Verification items for the finished model (mm, model axes). Face numbers are marked on the shaded views. A direction names the side the tool comes from. Round coordinates to 2 decimals unless told otherwise and drop trailing zeros. Order: outer loops, then holes, each group sorted by start corner. A loop starts at its lowest first (then second) coordinate and runs counter-clockwise, first axis right, second up.
```python
from build123d import *

# Parameters (mm, degrees)
F0_W     = 19.05
F0_H     = 69.85
F1_ANGLE = -270
F2_R     = 3.048
F3_W     = 34.798
F3_H     = 35.052
F4_ANGLE = 270
F5_R     = 3.048
F6_R     = 19.05
F7_DEPTH = 53.849
F8_R     = 6.35
F9_DEPTH = 19.051


with BuildPart() as f1:
    # F0 (on Right) → F1 (revolve)
    with BuildSketch(Plane.YZ):
        with Locations((9.525, 34.925)):
            Rectangle(F0_W, F0_H)
    revolve(axis=Axis((0, 9.525, 0), (0, 1, 0)), revolution_arc=F1_ANGLE)

    # F2
    f2_edges = [f1.edges().sort_by_distance(p)[0] for p in [
        (-49.391409, 0, -49.391409),
    ]]
    fillet(f2_edges, radius=F2_R)

    # F3 (on Right) → F4 (revolve)
    with BuildSketch(Plane.YZ):
        with Locations((-17.399, 17.526)):
            Rectangle(F3_W, F3_H)
    revolve(axis=Axis((0, -17.399, 0), (0, -1, 0)), revolution_arc=F4_ANGLE)

    # F5
    f5_edges = [f1.edges().sort_by_distance(p)[0] for p in [
        (-24.785507, -34.798, -24.785507),
        (-24.785507, 0, -24.785507),
    ]]
    fillet(f5_edges, radius=F5_R)

    # F6 (on face) → F7 (cut, through all)
    with BuildSketch(Plane.XZ.offset(34.798)):
        Circle(F6_R)
    extrude(amount=-F7_DEPTH, mode=Mode.SUBTRACT)

    # F8 (on Front) → F9 (cut, through all)
    with BuildSketch(Plane.XZ):
        with Locations((0, 53.848)):
            Circle(F8_R)
        with Locations((-53.848, 0)):
            Circle(F8_R)
        with Locations((0, -53.848)):
            Circle(F8_R)
        with Locations((53.848, 0)):
            Circle(F8_R)
    extrude(amount=-F9_DEPTH, mode=Mode.SUBTRACT)


solid = f1.part
```
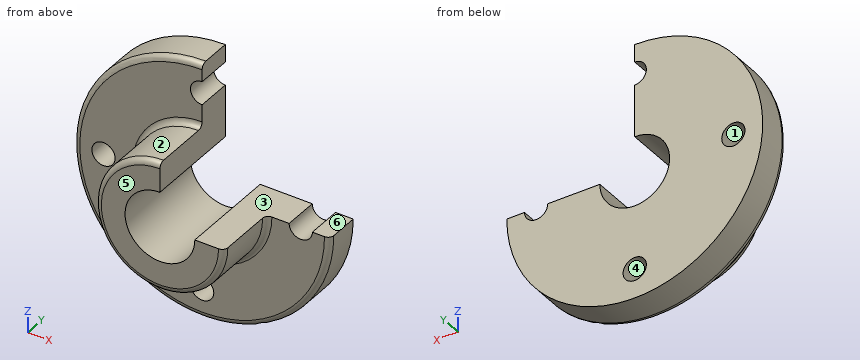
1) Go/stop test with flat-tipped pins: pin 1 Ø2 at (x, y) = (28.5, -7.5) entering from +Z; pin 2 Ø5 at (y, z) = (7, -34) entering from -X; pin 3 Ø5 at (y, z) = (10.5, 65.5) entering from +X. Record where each tip stops, or that it passes through.
2) Scan lines: probe 1 along X at (y, z) = (16.5, -2); probe 2 along Y at (x, z) = (28.5, -32); probe 3 along X at (y, z) = (-2.5, -10). Record each from-to range of solid material in increasing order.
3) Sectioned sample at A-A on y = 7.5. Record the cut outline in (x, z), then the cut area to 3 significant figures.
4) Sectioned sample at B-B on y = -23. Record the cut outline in (x, z), then the cut area to 3 significant figures.
5) Draft check along Z on the marked faces 4, 5 and 6. Enter one of: released by +Z, released by -Z, zero draft, split by the parting line, or undercut.
6) Tool access check on the marked faces 1, 2 and 3. Record the directions out of +Z, -Z, +X, -X, +Y, -Y that give a thin tool (end or side, any length) a straight path to the whole face; none if there is none.
Returned:
1. pin 1: stops at z = 0
1. pin 2: stops at x = -62.34
1. pin 3: stops at x = 0
2. probe 1: x = -69.82 to -59.87, -47.82 to -18.94, 18.94 to 47.82, 59.87 to 69.82
2. probe 2: y = 0 to 19.05
2. probe 3: x = -33.65 to -16.21, 16.21 to 33.65
3. outline: (0, 19.05) - (0, 47.5) arc R6.35 cw to (0, 60.2) - (0, 69.85) arc R69.85 ccw (long way) to (69.85, 0) - (60.2, 0) arc R6.35 cw to (47.5, 0) - (19.05, 0) arc R19.05 cw (long way) to start; hole circle Ø12.7 at (-53.85, 0); hole circle Ø12.7 at (0, -53.85)
3. area: 10,300 mm2
4. outline: (0, 19.05) - (0, 35.05) arc R35.05 ccw (long way) to (35.05, 0) - (19.05, 0) arc R19.05 cw (long way) to start
4. area: 2,040 mm2
5. face 4: undercut
5. face 5: zero draft
5. face 6: released by +Z
6. face 1: +Y, -Y
6. face 2: -Y
6. face 3: +Z, +X, +Y, -Y
